The figure shows three views and two pictorial views of one solid part (mm, origin at its lowest corner). Answer the questions. A direction names the side the tool comes from. Coordinates: 2 decimals unless noted, no trailing zeros. Order: outer loops, then holes, each group sorted by start corner. A loop starts at its lowest first (then second) coordinate and runs counter-clockwise, first axis right, second up. Notation, with made-up numbers: (-0.5, -6) - (16.5, -6) arc R20 cw to (16.5, 25) - close; hole circle Ø11 at (9.5, 11.25). An arc over 180 degrees is marked (long way). Answer as a JSON object with one key per item and string values. Group by question number.
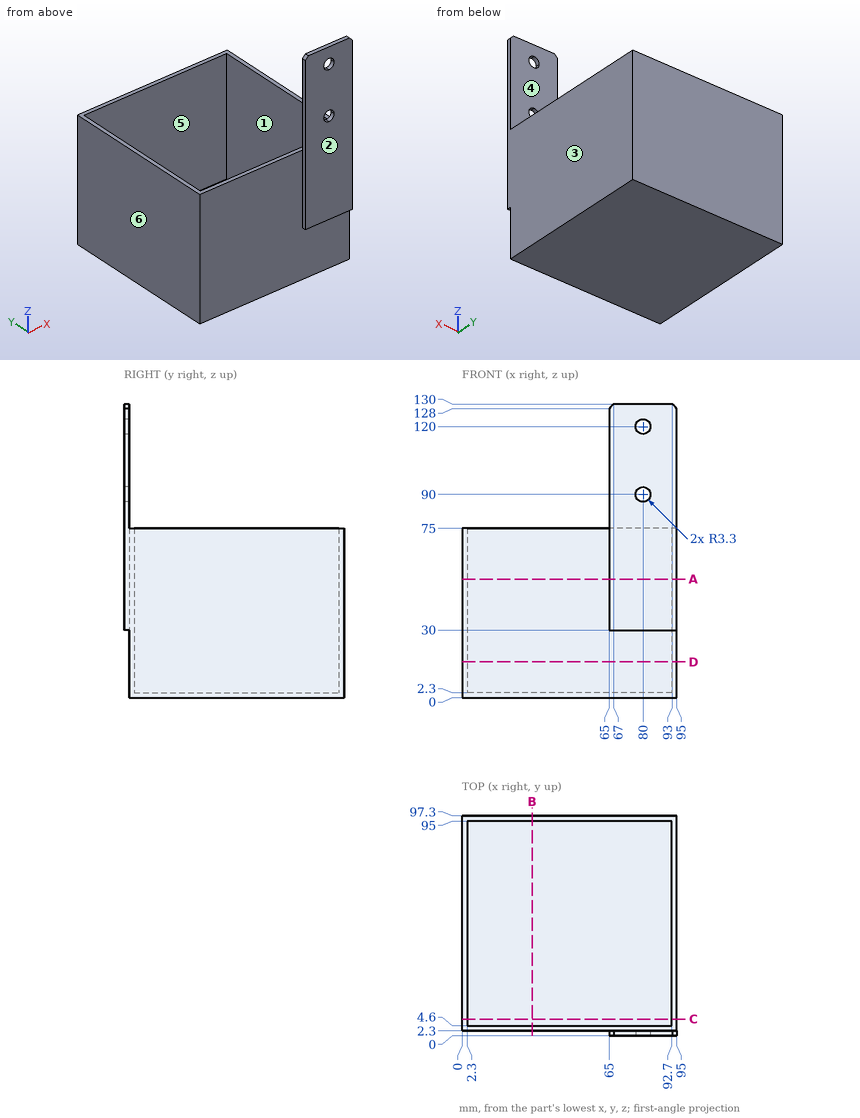
1. A cutting plane is placed at D-D on z = 16. Write down the section's boundary in (x, y), and give its area (3 significant figures).
2. A cutting plane is placed at A-A on z = 52.5. Write down the section's boundary in (x, y), and give its area (3 significant figures).
3. A cutting plane is placed at B-B on x = 31. Write down the section's boundary in (y, z), and give its area (3 significant figures).
4. Straight lines are drawn through the part: L1, parallel to Y at x = 28.5, z = 7.5; L2, parallel to X at y = 37, z = 43.5; L3, parallel to Z at x = 54.5, y = 85. For each, find the intervals that lie inside material, in ascending order.
5. A cutting plane is placed at C-C on y = 7.5. Write down the section's boundary in (x, z).
6. For the marked faces 1 and 2, determine the directions among +Z, -Z, +X, -X, +Y, -Y from which every point of the face is accessible in a straight line to the end or side of a thin tool.
7. For a pull along X with two mould halves and no side action, classify the marked faces 3, 4, 5 and 6 as pulls with the +X half, pulls with the -X half, needs draft (parallel to the pull), parting line crosses it, or undercut.
8. Given pin 1 (15 mm diameter, centred on x = 84.5, z = 95, fed in from +Y); pin 2 (1.5 mm diameter, centred on x = 31.5, y = 35.5, fed in from +Z); pin 3 (22.5 mm diameter, centred on x = 40, z = 23.5, fed in from -Y), each flat-ended and moving along its own axis, determine where each tip first touches the part or whether it passes through.
Derived:
{
 "1": {"outline": "(0, 2.3) - (95, 2.3) - (95, 97.3) - (0, 97.3) - close; hole (2.3, 4.6) - (92.7, 4.6) - (92.7, 95) - (2.3, 95) - close", "area": "853 mm2"},
 "2": {"outline": "(0, 2.3) - (65, 2.3) - (65, 0) - (95, 0) - (95, 97.3) - (0, 97.3) - close; hole (2.3, 4.6) - (92.7, 4.6) - (92.7, 95) - (2.3, 95) - close", "area": "922 mm2"},
 "3": {"outline": "(2.3, 0) - (97.3, 0) - (97.3, 75) - (95, 75) - (95, 2.3) - (4.6, 2.3) - (4.6, 75) - (2.3, 75) - close", "area": "553 mm2"},
 "4": {"L1": "y = 2.3 to 4.6, 95 to 97.3", "L2": "x = 0 to 2.3, 92.7 to 95", "L3": "z = 0 to 2.3"},
 "5": {"outline": "(0, 0) - (95, 0) - (95, 75) - (92.7, 75) - (92.7, 2.3) - (2.3, 2.3) - (2.3, 75) - (0, 75) - close"},
 "6": {"face 1": "+Z", "face 2": "+Z, -Z, +X, -X, -Y"},
 "7": {"face 3": "pulls with the +X half", "face 4": "needs draft", "face 5": "undercut", "face 6": "pulls with the -X half"},
 "8": {"pin 1": "stops at y = 2.3", "pin 2": "stops at z = 2.3", "pin 3": "stops at y = 2.3"}
}
